Here's how the part is built. I have some questions about the finished solid (model axes, mm). Face numbers are marked on the shaded views. Round coordinates to 2 decimals unless told otherwise and drop trailing zeros. Write each loop counter-clockwise with the first axis right and the second up, starting at its lowest first coordinate (ties: lowest second). Pieces come first, ordered by that corner, then holes. Notation, with made-up numbers: (64.5, 45.25) -> (79.5, 45.25) arc R31 cw to (79.5, 70.25) -> close; hole circle Ø10 at (34, -14.75). An arc over 180 degrees is marked (long way). Put each result on its own line as item: value. Start each with the question number.
1. We'd pull the mould along Y, two halves only. Please class the marked faces 1, 2 and 3: +Y half, -Y half, draft (parallel to the pull), parting line (faces both ways), or undercut.
2. I need wall thicknesses on probe 1 along Y at (x, z) = (64, 0); probe 2 along X at (y, z) = (-5, 15); probe 3 along Z at (x, y) = (40.5, 19). Which ranges of each line are inside material? Lowest first, please. Write a range as from..to.
3. For pin 1 (5 mm diameter, centred on y = 0.5, z = 20.5, fed in from +X); pin 2 (1 mm diameter, centred on y = -30.5, z = -0.5, fed in from +X); pin 3 (3 mm diameter, centred on y = -31, z = 0, fed in from -X) (3 decimals); pin 4 (2 mm diameter, centred on x = 68.5, y = -1, fed in from -Z), each with a flat end and sliding along its axis, tell me the tip position at first contact or that it passes through.
4. Suppose I cut it at A-A (x = 52). Please give me the cut outline in (y, z), then the cut area to 4 significant figures.
```python
from build123d import *

# Parameters (mm, degrees)
THICKEN1_T2                     = 2
SURFACE_EXTRUDE1_2_DEPTH        = 65
THICKEN2_T1                     = 2
BOSS_EXTRUDE2_REACH             = 83.701
BOSS_EXTRUDE2_END_MAJOR_RADIUS  = 15
BOSS_EXTRUDE2_END_MINOR_RADIUS  = 18
BOSS_EXTRUDE2_DIRECTION_2_DEPTH = 65
SKETCH5_R                       = 1
CUT_EXTRUDE2_DEPTH              = 65
SURFACE_EXTRUDE2_3_DEPTH        = 5
THICKEN3_T1                     = 1
SKETCH7_R                       = 5
CUT_EXTRUDE3_DEPTH              = 2


with BuildPart() as body_1:
    # Surface-Revolve1: a surface, the sketch's curves turned about an axis
    with BuildLine(Plane(origin=(0, 0, 0), x_dir=(1, 0, 0), z_dir=(0, 1, 0)), mode=Mode.PRIVATE) as surface_revolve1_1_path:
        Line((0, 0), (0, 15))
        ThreePointArc((0, 15), (5.857864376, 29.142135624), (20, 35))
    surface_revolve1_1 = Shell.revolve(surface_revolve1_1_path.wire(), 360, Axis((0, 0, 0), (1, 0, 0)))
    add(Solid.thicken(surface_revolve1_1, -THICKEN1_T2))

    # Surface-Extrude1: a surface, the sketch's curves swept straight by 65 mm
    with BuildLine(Plane(origin=(20, 0, 0), x_dir=(0, 0, -1), z_dir=(1, 0, 0)), mode=Mode.PRIVATE) as surface_extrude1_2_path:
        CenterArc((0, 0), 35, 0, 360)
    surface_extrude1_2 = Shell.extrude(surface_extrude1_2_path.wire(), (1 * SURFACE_EXTRUDE1_2_DEPTH, 0 * SURFACE_EXTRUDE1_2_DEPTH, 0 * SURFACE_EXTRUDE1_2_DEPTH))
    add(Solid.thicken(surface_extrude1_2, THICKEN2_T1))

    # Boss-Extrude2: up to this torus (the profile starts inside it)
    boss_extrude2_end = Plane(origin=(20, 0, 0), z_dir=(1, 0, 0)) * Torus(BOSS_EXTRUDE2_END_MAJOR_RADIUS, BOSS_EXTRUDE2_END_MINOR_RADIUS, mode=Mode.PRIVATE)
    # Sketch2 → Boss-Extrude2 (add, up to the surface)
    with BuildSketch(Plane(origin=(20, 0, 0), x_dir=(0, 0, -1), z_dir=(1, 0, 0)), mode=Mode.PRIVATE) as boss_extrude2_sk1:
        with BuildLine():
            Line((-2, 31), (-2, 33))
            Line((-2, 33), (2, 33))
            Line((2, 33), (2, 31))
            ThreePointArc((2, 31), (0, 29), (-2, 31))
        make_face()
    boss_extrude2_tool1 = extrude(boss_extrude2_sk1.sketch, amount=-BOSS_EXTRUDE2_REACH, mode=Mode.PRIVATE) & boss_extrude2_end
    add(boss_extrude2_tool1.solids().sort_by_distance((20, 31.1867, 0))[0])
    # Sketch2 → Boss-Extrude2 (add, up to the surface)
    with BuildSketch(Plane(origin=(20, 0, 0), x_dir=(0, 0, -1), z_dir=(1, 0, 0)), mode=Mode.PRIVATE) as boss_extrude2_sk2:
        with BuildLine():
            Line((-31, -2), (-33, -2))
            Line((-33, -2), (-33, 2))
            Line((-33, 2), (-31, 2))
            ThreePointArc((-31, 2), (-29, 0), (-31, -2))
        make_face()
    boss_extrude2_tool2 = extrude(boss_extrude2_sk2.sketch, amount=-BOSS_EXTRUDE2_REACH, mode=Mode.PRIVATE) & boss_extrude2_end
    add(boss_extrude2_tool2.solids().sort_by_distance((20, 0, 31.1867))[0])
    # Sketch2 → Boss-Extrude2 (add, up to the surface)
    with BuildSketch(Plane(origin=(20, 0, 0), x_dir=(0, 0, -1), z_dir=(1, 0, 0)), mode=Mode.PRIVATE) as boss_extrude2_sk3:
        with BuildLine():
            Line((2, -33), (2, -31))
            ThreePointArc((2, -31), (0, -29), (-2, -31))
            Line((-2, -31), (-2, -33))
            Line((-2, -33), (2, -33))
        make_face()
    boss_extrude2_tool3 = extrude(boss_extrude2_sk3.sketch, amount=-BOSS_EXTRUDE2_REACH, mode=Mode.PRIVATE) & boss_extrude2_end
    add(boss_extrude2_tool3.solids().sort_by_distance((20, -31.1867, 0))[0])
    # Sketch2 → Boss-Extrude2 (add, up to the surface)
    with BuildSketch(Plane(origin=(20, 0, 0), x_dir=(0, 0, -1), z_dir=(1, 0, 0)), mode=Mode.PRIVATE) as boss_extrude2_sk4:
        with BuildLine():
            Line((33, 2), (31, 2))
            ThreePointArc((31, 2), (29, 0), (31, -2))
            Line((31, -2), (33, -2))
            Line((33, -2), (33, 2))
        make_face()
    boss_extrude2_tool4 = extrude(boss_extrude2_sk4.sketch, amount=-BOSS_EXTRUDE2_REACH, mode=Mode.PRIVATE) & boss_extrude2_end
    add(boss_extrude2_tool4.solids().sort_by_distance((20, 0, -31.1867))[0])

    # Sketch2 → Boss-Extrude2 direction 2 (add)
    with BuildSketch(Plane(origin=(20, 0, 0), x_dir=(0, 0, -1), z_dir=(1, 0, 0))):
        with BuildLine():
            Line((-2, 31), (-2, 33))
            Line((-2, 33), (2, 33))
            Line((2, 33), (2, 31))
            ThreePointArc((2, 31), (0, 29), (-2, 31))
        make_face()
        with BuildLine():
            Line((-31, -2), (-33, -2))
            Line((-33, -2), (-33, 2))
            Line((-33, 2), (-31, 2))
            ThreePointArc((-31, 2), (-29, 0), (-31, -2))
        make_face()
        with BuildLine():
            Line((2, -33), (2, -31))
            ThreePointArc((2, -31), (0, -29), (-2, -31))
            Line((-2, -31), (-2, -33))
            Line((-2, -33), (2, -33))
        make_face()
        with BuildLine():
            Line((33, 2), (31, 2))
            ThreePointArc((31, 2), (29, 0), (31, -2))
            Line((31, -2), (33, -2))
            Line((33, -2), (33, 2))
        make_face()
    extrude(amount=BOSS_EXTRUDE2_DIRECTION_2_DEPTH)

    # Sketch5 → Cut-Extrude2 (cut)
    with BuildSketch(Plane(origin=(85, 0, 0), x_dir=(0, 0, -1), z_dir=(1, 0, 0))):
        with Locations((0, 31)):
            Circle(SKETCH5_R)
        with Locations((31, 0)):
            Circle(SKETCH5_R)
        with Locations((-31, 0)):
            Circle(SKETCH5_R)
        with Locations((0, -31)):
            Circle(SKETCH5_R)
    extrude(amount=-CUT_EXTRUDE2_DEPTH, mode=Mode.SUBTRACT)

    # Surface-Extrude2: a surface, the sketch's curves swept straight by 5 mm
    with BuildLine(Plane(origin=(85, 0, 0), x_dir=(0, 0, -1), z_dir=(1, 0, 0)), mode=Mode.PRIVATE) as surface_extrude2_3_path:
        CenterArc((0, 0), 35, 0, 360)
    surface_extrude2_3 = Shell.extrude(surface_extrude2_3_path.wire(), (1 * SURFACE_EXTRUDE2_3_DEPTH, 0 * SURFACE_EXTRUDE2_3_DEPTH, 0 * SURFACE_EXTRUDE2_3_DEPTH))
    add(Solid.thicken(surface_extrude2_3, THICKEN3_T1))

    # Sketch7 → Cut-Extrude3 (cut)
    with BuildSketch(Plane(origin=(0, 0, 0), x_dir=(0, 0, -1), z_dir=(1, 0, 0))):
        with Locations(Location((0, 0, 0), (0, 0, 180))):
            Circle(SKETCH7_R)
    extrude(amount=CUT_EXTRUDE3_DEPTH, mode=Mode.SUBTRACT)


solid = body_1.part
```
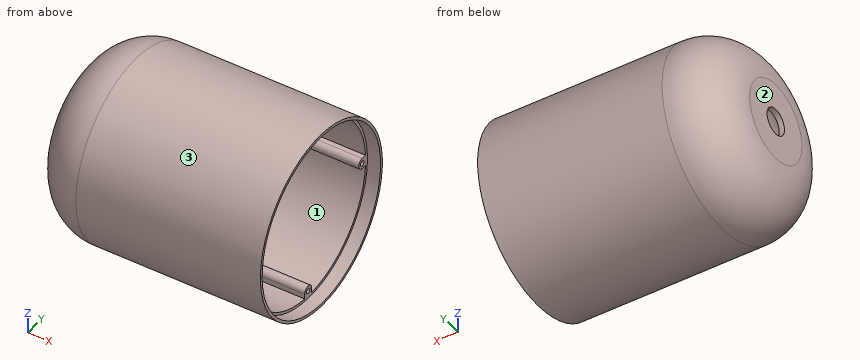
Verdict:
1. face 1: undercut
1. face 2: draft
1. face 3: parting line
2. probe 1: y = -35..-32, -30..-29, 29..30, 32..35
2. probe 2: x = 0.02..2.02
2. probe 3: z = -29.39..-26.98, 26.98..29.39
3. pin 1: stops at x = 3.88
3. pin 2: stops at x = 85
3. pin 3: stops at x = 6.225
3. pin 4: stops at z = -35
4. outline: circle Ø70 at (0, 0); hole (-32.94, -2) arc R33 ccw to (-2, -32.94) -> (-2, -31) arc R2 cw to (2, -31) -> (2, -32.94) arc R33 ccw to (32.94, -2) -> (31, -2) arc R2 cw to (31, 2) -> (32.94, 2) arc R33 ccw to (2, 32.94) -> (2, 31) arc R2 cw to (-2, 31) -> (-2, 32.94) arc R33 ccw to (-32.94, 2) -> (-31, 2) arc R2 cw to (-31, -2) -> close; hole circle Ø2 at (-31, 0); hole circle Ø2 at (0, -31); hole circle Ø2 at (0, 31); hole circle Ø2 at (31, 0)
4. area: 471.5 mm^2
